Design review of the part shown in the three views and the two pictorial views. Dimensions are in mm from the part's minimum x, y and z. A direction names the side the tool comes from. Round coordinates to 2 decimals unless told otherwise and drop trailing zeros. Loops run counter-clockwise (first coordinate to the right, second up) from the corner with the lowest first, then second, coordinate; pieces in that order, holes last. Notation, with made-up numbers: M -32,-22.75 L -9,-22.75 A18 cw -9,6.25 Z; hole C 72,-2.75 d9. An arc over 180 degrees is marked long. Return JSON: item names as keys, results as strings. Group by question number.
Q1. Consider section A-A (x = 1.5). State the section outline as (y, z) points, and give its area (3 significant figures).
Q2. Draft analysis for pull direction Y (two halves, no side actions). For the marked faces 3, 4, 5 and 6, state which applies: pulls with the +Y half, pulls with the -Y half, needs draft (parallel to the pull), parting line crosses it, or undercut.
Q3. To check wall thickness, follow line 1 along Y through (x, z) = (1.2, 2.8); line 2 along Z through (x, y) = (0.6, 7.25); line 3 along Z through (x, y) = (2.55, 3.5). State the ranges of each line that lie inside material, in increasing order.
Q4. Consider section B-B (z = 1.5). State the section outline as (x, y) points, and give its area (3 significant figures).
Q5. Consider section C-C (y = 8.5). State the section outline as (x, z) points, and give its area (3 significant figures).
Q6. Consider section D-D (y = 4.5). State the section outline as (x, z) points, and give its area (3 significant figures).
Q7. For the marked faces 1 and 2, list the 3-axis set-ups (+Z, -Z, +X, -X, +Y, -Y) from which the entire face can be reached by the end or side of a thin tool; tool diameter is ignored.
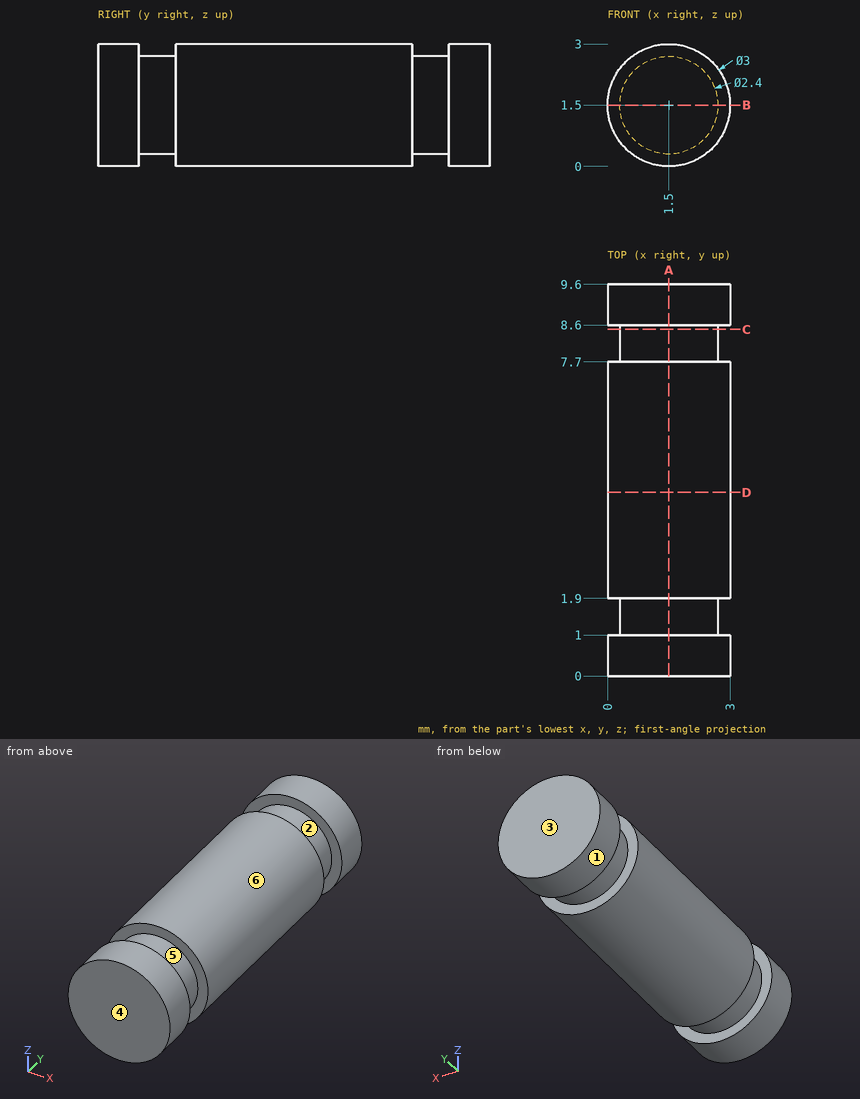
Values:
{
 "1": {"outline": "M 0,0 L 1,0 L 1,0.3 L 1.9,0.3 L 1.9,0 L 7.7,0 L 7.7,0.3 L 8.6,0.3 L 8.6,0 L 9.6,0 L 9.6,3 L 8.6,3 L 8.6,2.7 L 7.7,2.7 L 7.7,3 L 1.9,3 L 1.9,2.7 L 1,2.7 L 1,3 L 0,3 Z", "area": "27.7 mm2"},
 "2": {"face 3": "pulls with the +Y half", "face 4": "pulls with the -Y half", "face 5": "undercut", "face 6": "needs draft"},
 "3": {"line 1": "y = 0 to 1, 1.9 to 7.7, 8.6 to 9.6", "line 2": "z = 0.3 to 2.7", "line 3": "z = 0.43 to 2.57"},
 "4": {"outline": "M 0,0 L 3,0 L 3,1 L 2.7,1 L 2.7,1.9 L 3,1.9 L 3,7.7 L 2.7,7.7 L 2.7,8.6 L 3,8.6 L 3,9.6 L 0,9.6 L 0,8.6 L 0.3,8.6 L 0.3,7.7 L 0,7.7 L 0,1.9 L 0.3,1.9 L 0.3,1 L 0,1 Z", "area": "27.7 mm2"},
 "5": {"outline": "C 1.5,1.5 d2.4", "area": "4.52 mm2"},
 "6": {"outline": "C 1.5,1.5 d3", "area": "7.07 mm2"},
 "7": {"face 1": "+Y, -Y", "face 2": "none"}
}
